Work out the finished part from the listing and answer in its coordinate system (mm). A direction names the side the tool comes from. Give positions to 0.01 mm unless a question says otherwise; leave off trailing zeros. Order: outer loops, then holes, each group sorted by start corner. A loop starts at its lowest first (then second) coordinate and runs counter-clockwise, first axis right, second up. Notation, with made-up numbers: (-7.5, 16.25) -> (43.5, 16.25) arc R11 cw to (43.5, 36.25) -> close; hole circle Ø4 at (1, -8). An arc over 180 degrees is marked (long way). Use a Markdown table: item, result. Add a question column.
Autodesk Inventor part; units mm, degrees
ref_plane "YZ Plane" through (0, 0, 0) normal (1, 0, 0) x (0, 1, 0)
ref_plane "XZ Plane" through (0, 0, 0) normal (0, 1, 0) x (-1, 0, 0)
ref_plane "XY Plane" through (0, 0, 0) normal (0, 0, 1) x (1, 0, 0)
sketch "Sketch1" plane through (0, 0, 0) normal (0, 0, 1) x (1, 0, 0)
  line L0 (-14.3446, 13.462) -> (14.3446, 13.462)
  line L1 (14.3446, 13.462) -> (14.3446, -13.462)
  line L2 (14.3446, -13.462) -> (-14.3446, -13.462)
  line L3 (-14.3446, -13.462) -> (-14.3446, 13.462)
  line L4 (-14.3446, 13.462) -> (14.3446, -13.462) construction
  line L5 (14.3446, 13.462) -> (-14.3446, -13.462) construction
  point P0 (0, 0)
  dimension "d0" = 28.6893
  dimension "d1" = 26.924
ref_plane "Work Plane1" through (0, 0, 0) normal (0, 0, -1) x (-1, 0, 0)
sketch "Sketch2" plane through (0, 0, 0) normal (0, 0, -1) x (-1, 0, 0)
  circle A0 centre (0, 0) radius 25.4
  dimension "d4" = 50.8
extrude "Extrusion2" add sketch "Sketch2" against normal blind 12.7
extrude "Extrusion3" cut sketch "Sketch1" along normal through all
sketch "Sketch3" plane through (0, 0, 0) normal (0, 0, 1) x (1, 0, 0)
  line L0 (-14.3446, -13.462) -> (14.3446, -13.462)
  line L1 (-14.3446, 13.462) -> (-14.3446, -13.462)
  line L2 (14.3446, 13.462) -> (-14.3446, 13.462)
  line L3 (14.3446, -13.462) -> (14.3446, 13.462)
  line L4 (-14.3446, 13.462) -> (-14.3446, -13.462)
  line L5 (-14.3446, -13.462) -> (14.3446, -13.462)
  line L6 (14.3446, -13.462) -> (14.3446, 13.462)
  line L7 (14.3446, 13.462) -> (-14.3446, 13.462)
  circle A0 centre (0, 0) radius 25.4
  line L8 (-35.56, 0) -> (35.56, 0)
  line L9 (0, -35.56) -> (0, 35.56)
  line L10 (14.3446, 13.462) -> (-14.3446, 13.462)
  line L11 (-14.3446, -13.462) -> (14.3446, -13.462)
  line L12 (14.3446, -13.462) -> (14.3446, 13.462)
  line L13 (14.3446, 13.462) -> (-14.3446, 13.462)
  line L14 (-14.3446, 13.462) -> (-14.3446, -13.462)
  line L15 (-14.3446, -13.462) -> (14.3446, 13.462) construction
  line L16 (14.3446, -13.462) -> (-14.3446, 13.462) construction
  line L17 (14.3446, 13.462) -> (-14.3446, 13.462)
  line L18 (-14.3446, -13.462) -> (14.3447, -13.462)
  line L19 (14.3447, -13.462) -> (14.3446, 13.462)
  line L20 (14.3446, 13.462) -> (-14.3446, 13.462)
  line L21 (-14.3446, 13.462) -> (-14.3446, -13.462)
  line L22 (-14.3446, -13.462) -> (14.3446, 13.462) construction
  line L23 (14.3447, -13.462) -> (-14.3446, 13.462) construction
  line L24 (14.3446, -13.462) -> (14.3446, 13.462)
extrude "Extrusion4" add sketch "Sketch3" along normal blind 0.1524 contours L1 L8 L9 L0 | L9 L8 L3 L0 | L1 L2 L9 L8 | L9 L2 L3 L8
pattern_linear "Rectangular Pattern1" [suppressed]
sketch "Sketch4" plane through (0, 0, 0) normal (0, 0, 1) x (1, 0, 0)
  circle A0 centre (0, 0) radius 25.4
  line L0 (-35.56, 0) -> (35.56, 0)
  line L1 (0, -35.56) -> (0, 35.56)
  line L2 (-14.3446, -13.462) -> (14.3446, -13.462)
  line L3 (13.5954, 13.462) -> (13.5954, -13.462)
  line L4 (-12.1856, -13.462) -> (13.5954, -13.462)
  line L5 (13.5954, -13.462) -> (13.5954, -0.254)
  line L6 (13.5954, -0.254) -> (-12.1857, -0.254)
  line L7 (-12.1857, -0.254) -> (-12.1856, -13.462)
  line L8 (13.2144, 13.462) -> (13.5954, 13.462)
  line L9 (10.6744, 13.462) -> (11.0554, 13.462)
  line L10 (8.1344, 13.462) -> (8.5154, 13.462)
  line L11 (5.5944, 13.462) -> (5.9754, 13.462)
  line L12 (3.0544, 13.462) -> (3.4354, 13.462)
  line L13 (0.5144, 13.462) -> (0.8954, 13.462)
  line L14 (-2.0256, 13.462) -> (-1.6446, 13.462)
  line L15 (-4.5656, 13.462) -> (-4.1846, 13.462)
  line L16 (-7.1056, 13.462) -> (-6.7246, 13.462)
  line L17 (-9.6456, 13.462) -> (-9.2646, 13.462)
  line L18 (-12.1856, 13.462) -> (-11.8046, 13.462)
  line L19 (-12.1856, 13.462) -> (-11.8046, 13.462)
  line L20 (-12.1856, 13.462) -> (13.5954, 13.462)
  line L21 (13.5954, 13.462) -> (13.5954, 0.254)
  line L22 (13.5954, 0.254) -> (-12.1857, 0.254)
  line L23 (-12.1857, 0.254) -> (-12.1856, 13.462)
  point P0 (-11.8046, -13.462)
  dimension "d15" = 0.254
extrude "Extrusion5" [suppressed]
sketch "Sketch5" plane through (0, 0, 0) normal (0, 0, -1) x (-1, 0, 0)
  circle A0 centre (0, 0) radius 25.4
  line L0 (35.56, 0) -> (-35.56, 0)
  line L1 (0, -35.56) -> (0, 35.56)
  circle A1 centre (11.9952, -2.794) radius 0.5
  point P0 (11.9952, -0.254)
  dimension "d18" = 1
extrude "Extrusion6" [suppressed]
pattern_linear "Rectangular Pattern2" [suppressed]
mirror "Mirror1" [suppressed]
sketch "Sketch6" plane through (0, 0, 0) normal (0, 0, -1) x (-1, 0, 0)
  point P0 (0, 0)
equation "\"BendRadius\" = Thickness"
equation "\"BendReliefWidth\" = Thickness"
equation "\"BendReliefDepth\" = 0.5 * Thickness"
equation "\"CornerReliefSize\" = 4 * Thickness"
equation "\"MinimumRemnant\" = 2 * Thickness"
equation "\"TransitionRadius\" = BendRadius"
equation "\"JacobiRadiusSize\" = BendRadius"
equation "\"GapSize\" = Thickness"
properties part number "_3DPrint"
1) The part is cut by section C-C, the plane x = 0. Determine the outline of the cut face in (y, z), then the cut area to 3 significant figures.
2) The part is cut by section B-B, the plane z = 5. Determine the outline of the cut face in (x, y), then the cut area to 3 significant figures.
3) Straight lines are drawn through the part: line 1 (Y direction, x = 9, z = 2.25); line 2 (X direction, y = -7, z = 8.75); line 3 (Y direction, x = -5.5, z = 9). For each, find the intervals that lie inside material, in ascending order.
4) Which of the six approach directions +Z, -Z, +X, -X, +Y, -Y give full straight-line access (tool end or side, diameter ignored) to faces 5 (the flat face through (0, 13.462, 6)), 6 (the flat face through (0, 0, 0))?
5) The part is cut by section D-D, the plane x = -16. Determine the outline of the cut face in (y, z).
6) Determine the mould class of faces 1 (the flat face through (-14.345, 0, 6)), 2 (the flat face through (0, -13.462, 6)), 3 (the flat face through (0, -17, 12.7)), 4 (the cylindrical face through (5.506, -24.796, 6.261)) for opening direction X: released by +X, released by -X, zero draft, split by the parting line, or undercut.
7) The part is cut by section A-A, the plane y = 0. Determine the outline of the cut face in (x, z).
8) Flat-ended cylindrical pins translate along their axes: pin 1 (1 mm diameter, centred on y = -3, z = 2.5, fed in from -X); pin 2 (4 mm diameter, centred on y = -12, z = 8, fed in from -X); pin 3 (6 mm diameter, centred on x = 2, z = 6, fed in from +Y). Find the tip coordinate at first contact, or state that the pin passes through.
A:
| question | item | result |
|---|---|---|
| 1 | outline | (-25.4, 0) -> (25.4, 0) -> (25.4, 12.7) -> (13.46, 12.7) -> (13.46, 0.15) -> (-13.46, 0.15) -> (-13.46, 12.7) -> (-25.4, 12.7) -> close |
| 1 | area | 307 mm^2 |
| 2 | outline | circle Ø50.8 at (0, 0); hole (-14.34, -13.46) -> (14.34, -13.46) -> (14.34, 13.46) -> (-14.34, 13.46) -> close |
| 2 | area | 1,250 mm^2 |
| 3 | line 1 | -23.75 to -13.46, 13.46 to 23.75 |
| 3 | line 2 | -24.42 to -14.34, 14.34 to 24.42 |
| 3 | line 3 | -24.8 to -13.46, 13.46 to 24.8 |
| 4 | face 5 | +Z |
| 4 | face 6 | -Z, +X, -X, +Y, -Y |
| 5 | outline | (-19.73, 0) -> (19.73, 0) -> (19.73, 12.7) -> (-19.73, 12.7) -> close |
| 6 | face 1 | undercut |
| 6 | face 2 | undercut |
| 6 | face 3 | zero draft |
| 6 | face 4 | split by the parting line |
| 7 | outline | (-25.4, 0) -> (25.4, 0) -> (25.4, 12.7) -> (14.34, 12.7) -> (14.34, 0.15) -> (-14.34, 0.15) -> (-14.34, 12.7) -> (-25.4, 12.7) -> close |
| 8 | pin 1 | x = -25.28 |
| 8 | pin 2 | x = -23.35 |
| 8 | pin 3 | y = 25.4 |
